from build123d import *

# Parameters (mm, degrees)
SKETCH1_W                      = 75
SKETCH1_H                      = 40
BOSS_EXTRUDE1_DEPTH            = 5
SKETCH3_W                      = 35
SKETCH3_H                      = 40
BOSS_EXTRUDE2_DEPTH            = 15
FILLET1_R                      = 2
FILLET2_R                      = 2
M5_CLEARANCE_HOLE1_D           = 5.5
M5_CLEARANCE_HOLE1_CSINK_D     = 5.55
M5_CLEARANCE_HOLE1_CSINK_ANGLE = 90


with BuildPart() as part:
    # Sketch1 → Boss-Extrude1 (new body)
    with BuildSketch(Plane(origin=(0, 0, 0), x_dir=(1, 0, 0), z_dir=(0, 1, 0))):
        Rectangle(SKETCH1_W, SKETCH1_H)
    extrude(amount=BOSS_EXTRUDE1_DEPTH)

    # Sketch3 → Boss-Extrude2 (add)
    with BuildSketch(Plane(origin=(0, 5, 0), x_dir=(1, 0, 0), z_dir=(0, 1, 0))):
        Rectangle(SKETCH3_W, SKETCH3_H)
    extrude(amount=BOSS_EXTRUDE2_DEPTH)

    # Fillet1
    fillet1_edges = [part.edges().sort_by_distance(p)[0] for p in [
        (-37.5, 2.5, -20),
        (-37.5, 2.5, 20),
        (37.5, 2.5, 20),
        (37.5, 2.5, -20),
    ]]
    fillet(fillet1_edges, radius=FILLET1_R)

    # Fillet2
    fillet2_edges = [part.edges().sort_by_distance(p)[0] for p in [
        (17.5, 12.5, 20),
        (17.5, 12.5, -20),
        (-17.5, 12.5, -20),
        (-17.5, 12.5, 20),
        (17.5, 20, 0),
        (0, 20, -20),
        (-17.5, 20, 0),
        (0, 20, 20),
    ]]
    fillet(fillet2_edges, radius=FILLET2_R)

    # M5 Clearance Hole1 (through all)
    with Locations(Plane(origin=(-27.5, 0, 10), x_dir=(0, 0, -1), z_dir=(0, -1, 0))):
        with Locations((0, 0), (20, 0)):
            m5_clearance_hole1 = CounterSinkHole(M5_CLEARANCE_HOLE1_D / 2, M5_CLEARANCE_HOLE1_CSINK_D / 2, counter_sink_angle=M5_CLEARANCE_HOLE1_CSINK_ANGLE)

    # Mirror1: M5 Clearance Hole1 across plane
    add(m5_clearance_hole1.mirror(Plane(origin=(0, 0, 0), x_dir=(0, 0, 1), z_dir=(1, 0, 0))), mode=Mode.SUBTRACT)


solid = part.part
For this review, take the finished solid that the model builds, in its own axes (mm). A direction names the side the tool comes from. Give positions to 0.01 mm unless a question says otherwise; leave off trailing zeros. Order: outer loops, then holes, each group sorted by start corner. A loop starts at its lowest first (then second) coordinate and runs counter-clockwise, first axis right, second up. Notation, with made-up numbers: (33, 61) - (50, 61) arc R29 cw to (50, 83) - close; hole circle Ø8 at (-9.75, -6). An arc over 180 degrees is marked (long way). Answer as a JSON object with one key per item and string values. Group by question number.
Item 1: Wall thickness on line 1 along X through (y, z) = (1.6, 10); line 2 along Y through (x, z) = (-32, 10); line 3 along X through (y, z) = (7.75, 5): over which ranges is each line inside the solid? List them lowest first.
Item 2: Take a section at D-D on z = 4.5. Give the boundary of the cut face in (x, y).
Item 3: Machinability: for faces 4 (the flat face through (17.5, 11, 0)), 5 (the flat face through (-17.5, 11, 0)), 6 (the cylindrical face through (16.9, 11.59, 19.43)), which of the approach directions +Z, -Z, +X, -X, +Y, -Y give a long, thin tool a straight path to every point of the face, cutting with its end or side? Answer none if there is none.
Item 4: Draft analysis for pull direction Z (two halves, no side actions). For faces 1 (the flat face through (0, 20, 0)), 2 (the cylindrical face through (-24.773, 2.547, 9.642)), 3 (the flat face through (0, 7, -20)), state which applies: pulls with the +Z half, pulls with the -Z half, needs draft (parallel to the pull), parting line crosses it, or undercut.
Item 5: Take a section at A-A on z = 10. Give the boundary of the cut face in (x, y) (3 decimals), and give its area (3 significant figures).
Item 6: Clearance check with flat-ended pins moving along their axes: pin 1 Ø11 at (x, z) = (30.5, 2) entering from +Y; pin 2 Ø3.5 at (x, z) = (-27.5, 10) entering from +Y; pin 3 Ø1.5 at (y, z) = (9.5, -14.5) entering from +X; pin 4 Ø8 at (x, z) = (-7.5, -13.5) entering from -Y. State where each tip first meets the part, or that it passes through.
Item 7: Take a section at B-B on x = 27.5. Give the boundary of the cut face in (y, z) (3 decimals), and give its area (3 significant figures).
Item 8: Take a section at C-C on y = 2.5. Give the boundary of the cut face in (x, z), and give its area (3 significant figures).
Reported:
{
 "1": {"line 1": "-37.5 to -30.25, -24.75 to 24.75, 30.25 to 37.5", "line 2": "0 to 5", "line 3": "-17.5 to 17.5"},
 "2": {"outline": "(-37.5, 0) - (37.5, 0) - (37.5, 5) - (17.5, 5) - (17.5, 18) arc R2 ccw to (15.5, 20) - (-15.5, 20) arc R2 ccw to (-17.5, 18) - (-17.5, 5) - (-37.5, 5) - close"},
 "3": {"face 4": "+Z, -Z, +X, +Y", "face 5": "+Z, -Z, -X, +Y", "face 6": "+Z, +X, +Y"},
 "4": {"face 1": "needs draft", "face 2": "undercut", "face 3": "pulls with the -Z half"},
 "5": {"outline": "(-37.5, 0) - (-30.275, 0) - (-30.25, 0.025) - (-30.25, 5) - (-37.5, 5) - close; (-24.75, 0.025) - (-24.725, 0) - (24.725, 0) - (24.75, 0.025) - (24.75, 5) - (17.5, 5) - (17.5, 18) arc R2 ccw to (15.5, 20) - (-15.5, 20) arc R2 ccw to (-17.5, 18) - (-17.5, 5) - (-24.75, 5) - close; (30.25, 0.025) - (30.275, 0) - (37.5, 0) - (37.5, 5) - (30.25, 5) - close", "area": "843 mm^2"},
 "6": {"pin 1": "y = 5", "pin 2": "through", "pin 3": "x = 17.5", "pin 4": "y = 0"},
 "7": {"outline": "(0, -20) - (5, -20) - (5, -12.75) - (0.025, -12.75) - (0, -12.775) - close; (0, -7.225) - (0.025, -7.25) - (5, -7.25) - (5, 7.25) - (0.025, 7.25) - (0, 7.225) - close; (0, 12.775) - (0.025, 12.75) - (5, 12.75) - (5, 20) - (0, 20) - close", "area": "145 mm^2"},
 "8": {"outline": "(-37.5, -18) arc R2 ccw to (-35.5, -20) - (35.5, -20) arc R2 ccw to (37.5, -18) - (37.5, 18) arc R2 ccw to (35.5, 20) - (-35.5, 20) arc R2 ccw to (-37.5, 18) - close; hole circle Ø5.5 at (-27.5, -10); hole circle Ø5.5 at (-27.5, 10); hole circle Ø5.5 at (27.5, -10); hole circle Ø5.5 at (27.5, 10)", "area": "2,900 mm^2"}
}
